Work out the finished part from the listing and answer in its coordinate system (mm). Give positions to 0.01 mm unless a question says otherwise; leave off trailing zeros. Loops run counter-clockwise (first coordinate to the right, second up) from the corner with the lowest first, then second, coordinate; pieces in that order, holes last. Notation, with made-up numbers: M 43.25,14 L 73.25,14 A17 cw 73.25,29 Z; hole C 88.25,-1.5 d2. An arc over 180 degrees is marked long. Write item = value, one per line. Start each with the question number.
1. Section D-D on z = -14 is taken. Determine the outline of the cut face in (x, y) (1 decimal), plus the area to 3 significant figures.
2. Flat-ended cylindrical pins translate along their axes: pin 1 Ø1.5 at (x, y) = (9, 2) entering from +Z; pin 2 Ø2.5 at (x, z) = (20.25, -14) entering from +Y; pin 3 Ø1.6 at (y, z) = (2, 5.5) entering from +X; pin 4 Ø1 at (y, z) = (2.5, -31.5) entering from +X. Find the tip coordinate at first contact, or state that the pin passes through.
3. Section B-B on x = 20.25 is taken. Determine the outline of the cut face in (y, z) (1 decimal).
4. Section C-C on y = 0.65 is taken. Give the number of separate pieces and of enclosed holes in the cut face, plus the area to 3 significant figures.
5. Consider L1, parallel to X at y = 2.4, z = -5; L2, parallel to X at y = 1.7, z = -44; L3, parallel to Z at x = 25.5, y = 0.7. Determine where each line is inside the solid, lowest interval first. Write a range as [from, to].
6. Section A-A on z = -5 is taken. Determine the outline of the cut face in (x, y) (3 decimals).
```python
from build123d import *

# Parameters (mm, degrees)
CROQUIS1_R              = 1.5875
SALIENTE_EXTRUIR1_DEPTH = 3.175
CROQUIS2_R              = 1.5875
CORTAR_EXTRUIR1_DEPTH   = 3.175
CROQUIS3_W              = 30
CROQUIS3_H              = 12.5
SALIENTE_EXTRUIR2_DEPTH = 3.175


with BuildPart() as part:
    # Croquis1 → Saliente-Extruir1 (new body)
    with BuildSketch(Plane(origin=(0, 0, 0), x_dir=(1, 0, 0), z_dir=(0, 1, 0))):
        with BuildLine():
            Line((8.713785816, 43.568929081), (0, 0))
            Line((0, 0), (60, 0))
            Line((60, 0), (51.286214184, 43.568929081))
            ThreePointArc((51.286214184, 43.568929081), (48.513480023, 48.186737131), (43.441568778, 50))
            Line((43.441568778, 50), (16.558431222, 50))
            ThreePointArc((16.558431222, 50), (11.486519977, 48.186737131), (8.713785816, 43.568929081))
        make_face()
        with Locations(Location((39.75, 14, 0), (0, 0, 270))):
            Circle(CROQUIS1_R, mode=Mode.SUBTRACT)
        with Locations(Location((20.25, 14, 0), (0, 0, 270))):
            Circle(CROQUIS1_R, mode=Mode.SUBTRACT)
        with Locations(Location((24.75, 44, 0), (0, 0, 270))):
            Circle(CROQUIS1_R, mode=Mode.SUBTRACT)
        with Locations(Location((35.25, 44, 0), (0, 0, 270))):
            Circle(CROQUIS1_R, mode=Mode.SUBTRACT)
    extrude(amount=SALIENTE_EXTRUIR1_DEPTH)

    # Croquis2 → Cortar-Extruir1 (cut)
    with BuildSketch(Plane(origin=(0, 3.175, 0), x_dir=(1, 0, 0), z_dir=(0, 1, 0))):
        with Locations(Location((6.099019514, 5, 0), (0, 0, 270))):
            Circle(CROQUIS2_R)
        with Locations(Location((53.900980486, 5, 0), (0, 0, 270))):
            Circle(CROQUIS2_R)
        with BuildLine():
            Line((53.900980486, 0), (60, 0))
            Line((60, 0), (58.803883865, 5.980580676))
            ThreePointArc((58.803883865, 5.980580676), (57.767691193, 1.830055472), (53.900980486, 0))
        make_face()
        with BuildLine():
            Line((1.196116135, 5.980580676), (0, 0))
            Line((0, 0), (6.099019514, 0))
            ThreePointArc((6.099019514, 0), (2.232308807, 1.830055472), (1.196116135, 5.980580676))
        make_face()
    extrude(amount=-CORTAR_EXTRUIR1_DEPTH, mode=Mode.SUBTRACT)

    # Croquis3 → Saliente-Extruir2 (add)
    with BuildSketch(Plane(origin=(0, 3.175, 0), x_dir=(1, 0, 0), z_dir=(0, 1, 0))):
        with Locations((30, -6.25)):
            Rectangle(CROQUIS3_W, CROQUIS3_H)
    extrude(amount=-SALIENTE_EXTRUIR2_DEPTH)


solid = part.part
```
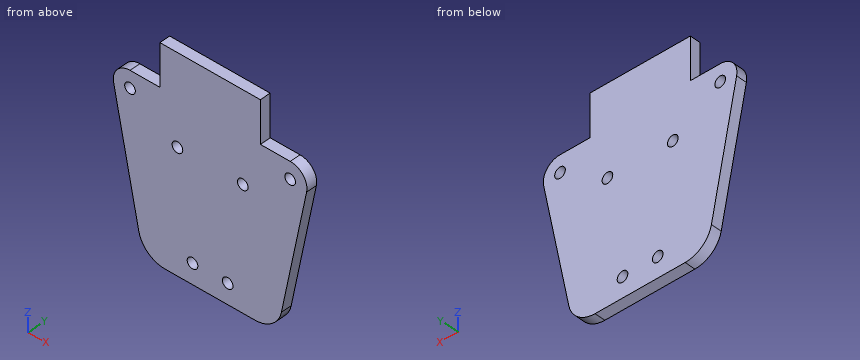
Verdict:
q1.outline = M 2.8,0 L 18.7,0 L 18.7,3.2 L 2.8,3.2 Z; M 21.8,0 L 38.2,0 L 38.2,3.2 L 21.8,3.2 Z; M 41.3,0 L 57.2,0 L 57.2,3.2 L 41.3,3.2 Z
q1.area = 153 mm2
q2.pin_1 = 0
q2.pin_2 = through
q2.pin_3 = 45
q2.pin_4 = 53.8
q3.outline = M 0,-50 L 3.2,-50 L 3.2,-15.6 L 0,-15.6 Z; M 0,-12.4 L 3.2,-12.4 L 3.2,12.5 L 0,12.5 Z
q4.separate_pieces = 1
q4.enclosed_holes = 6
q4.area = 2,790 mm2
q5.L1 = [1.1, 4.51], [7.69, 52.31], [55.49, 58.9]
q5.L2 = [8.81, 23.16], [26.34, 33.66], [36.84, 51.19]
q5.L3 = [-50, -45.4], [-42.6, 12.5]
q6.outline = M 1.099,0 L 4.512,0 L 4.512,3.175 L 1.099,3.175 Z; M 7.687,0 L 52.313,0 L 52.313,3.175 L 7.687,3.175 Z; M 55.488,0 L 58.901,0 L 58.901,3.175 L 55.488,3.175 Z
